For this review, take the finished solid that the model builds, in its own axes (mm). A direction names the side the tool comes from. Give positions to 0.01 mm unless a question says otherwise; leave off trailing zeros. Write each loop counter-clockwise with the first axis right and the second up, starting at its lowest first coordinate (ties: lowest second). Pieces come first, ordered by that corner, then holes.
1) We need section A-A on y = 1. Give the boundary of the cut face in (x, z), and give its area (3 significant figures).
2) Machinability: for faces 1 (the face through (125.556, -67, 2)), 2 (the face through (-121, 55.466, 2)), 3 (the face through (0, -40.914, 2)), 4 (the face through (121, -29.881, 2)), 5 (the face through (-41.016, 12, 2)), which of the approach directions +Z, -Z, +X, -X, +Y, -Y give a long, thin tool a straight path to every point of the face, cutting with its end or side? Answer none if there is none.
3) We need section B-B on x = 59. Give the boundary of the cut face in (y, z), and give its area (3 significant figures).
4) We need section D-D on x = -90. Give the boundary of the cut face in (y, z), and give its area (3 significant figures).
5) Wall thickness on line 1 along Y through (x, z) = (26.5, 0.55); line 2 along X through (y, z) = (39, 2.1); line 3 along Y through (x, z) = (-79.5, 2.9): over which ranges is each line inside the solid? List them lowest first.
6) We need section C-C on y = -59.5. Give the boundary of the cut face in (x, z), and give its area (3 significant figures).
7) Draft analysis for pull direction X (two halves, no side actions). For faces 6 (the face through (-115.712, 13, 2)), 7 (the face through (96.437, -75.828, 2.465)), 8 (the face through (41.016, 12, 2)), 9 (the face through (-98, -102.438, 2)), state which applies: pulls with the +X half, pulls with the -X half, needs draft (parallel to the pull), parting line crosses it, or undercut.
8) For P1, Ø1.5, axis at y = 8, z = 3, coming from the +X side, flat-tipped, find the tip position at first contact; note if it passes through.
from build123d import *

# Parameters (mm, degrees)
SKETCH1_R           = 2.153330351
SKETCH1_R_2         = 12.817442563
SKETCH1_W           = 33.838048367
SKETCH1_H           = 82.031632405
BOSS_EXTRUDE1_DEPTH = 5
SKETCH5_R           = 62
CUT_EXTRUDE3_DEPTH  = 5
SKETCH6_R           = 1.6
SKETCH6_R_2         = 2
CUT_EXTRUDE4_DEPTH  = 10
BOSS_EXTRUDE2_DEPTH = 5
CUT_EXTRUDE5_DEPTH  = 30


with BuildPart() as part:
    # Sketch1 → Boss-Extrude1 (new body)
    with BuildSketch(Plane.XY):
        with BuildLine():
            Line((125.53231807, 103.262634184), (91.381905468, 103.262634184))
            Line((91.381905468, 103.262634184), (77.913526918, 103.262634184))
            Line((77.913526918, 103.262634184), (36.253297751, 103.262634184))
            ThreePointArc((36.253297751, 103.262634184), (0, 93.454499378), (-36.253297751, 103.262634184))
            Line((-36.253297751, 103.262634184), (-77.913526918, 103.262634184))
            Line((-77.913526918, 103.262634184), (-91.381905468, 103.262634184))
            Line((-91.381905468, 103.262634184), (-125.53231807, 103.262634184))
            Line((-125.53231807, 103.262634184), (-125.54905558, 83.520799446))
            Line((-125.54905558, 83.520799446), (-125.554160174, 70.087177042))
            Line((-125.554160174, 70.087177042), (-125.554470078, 55.465919402))
            Line((-125.554470078, 55.465919402), (-115.83891891, 55.465919402))
            Line((-115.83891891, 55.465919402), (-115.711941884, 55.465919402))
            Line((-115.711941884, 55.465919402), (-115.711941884, 55.338942376))
            Line((-115.711941884, 55.338942376), (-115.711941884, -29.754151955))
            Line((-115.711941884, -29.754151955), (-115.711941884, -29.88112898))
            Line((-115.711941884, -29.88112898), (-115.83891891, -29.88112898))
            Line((-115.83891891, -29.88112898), (-125.555737773, -29.88112898))
            Line((-125.555737773, -29.88112898), (-125.555737773, -59.42445768))
            Line((-125.555737773, -59.42445768), (-125.555737773, -72.892836229))
            Line((-125.555737773, -72.892836229), (-125.555737773, -102.437610833))
            Line((-125.555737773, -102.437610833), (-101.198740966, -102.437610833))
            Line((-101.198740966, -102.437610833), (-87.730362416, -102.437610833))
            Line((-87.730362416, -102.437610833), (-70.522775483, -102.437610833))
            Line((-70.522775483, -102.437610833), (-52.513332124, -71.244339919))
            Line((-52.513332124, -71.244339919), (-47.927289793, -63.301081597))
            Line((-47.927289793, -63.301081597), (-35.002036695, -40.91388653))
            Line((-35.002036695, -40.91388653), (-5.325262411, -40.91388653))
            Line((-5.325262411, -40.91388653), (5.324834587, -40.91388653))
            Line((5.324834587, -40.91388653), (35.002036695, -40.91388653))
            Line((35.002036695, -40.91388653), (47.927289793, -63.301081597))
            Line((47.927289793, -63.301081597), (52.513332124, -71.244339919))
            Line((52.513332124, -71.244339919), (70.522775483, -102.437610833))
            Line((70.522775483, -102.437610833), (87.730362416, -102.437610833))
            Line((87.730362416, -102.437610833), (101.198740966, -102.437610833))
            Line((101.198740966, -102.437610833), (125.555737773, -102.437610833))
            Line((125.555737773, -102.437610833), (125.555737773, -72.892113277))
            Line((125.555737773, -72.892113277), (125.555737773, -59.423734727))
            Line((125.555737773, -59.423734727), (125.555737773, -29.88112898))
            Line((125.555737773, -29.88112898), (115.83891891, -29.88112898))
            ThreePointArc((115.83891891, -29.88112898), (115.749132594, -29.843938271), (115.711941884, -29.754151955))
            Line((115.711941884, -29.754151955), (115.711941884, 55.338942376))
            ThreePointArc((115.711941884, 55.338942376), (115.749132594, 55.428728692), (115.83891891, 55.465919402))
            Line((115.83891891, 55.465919402), (125.554470078, 55.465919402))
            Line((125.554470078, 55.465919402), (125.554160387, 70.077114789))
            Line((125.554160387, 70.077114789), (125.549047054, 83.530856147))
            Line((125.549047054, 83.530856147), (125.53231807, 103.262634184))
        make_face()
        with Locations((-101.032414216, -82.661089892)):
            Circle(SKETCH1_R, mode=Mode.SUBTRACT)
        with Locations((-90.522111314, -64.456711263)):
            Circle(SKETCH1_R_2, mode=Mode.SUBTRACT)
        with Locations((-80.011808412, -46.252332635)):
            Circle(SKETCH1_R, mode=Mode.SUBTRACT)
        with Locations((80.011808412, -46.252332635)):
            Circle(SKETCH1_R, mode=Mode.SUBTRACT)
        with Locations((90.522111314, -64.456711263)):
            Circle(SKETCH1_R_2, mode=Mode.SUBTRACT)
        with Locations((101.032414216, -82.661089892)):
            Circle(SKETCH1_R, mode=Mode.SUBTRACT)
        with Locations((57.934840386, 12.792395211)):
            Rectangle(SKETCH1_W, SKETCH1_H, mode=Mode.SUBTRACT)
        with Locations((-57.934840386, 12.792395211)):
            Rectangle(SKETCH1_W, SKETCH1_H, mode=Mode.SUBTRACT)
    extrude(amount=BOSS_EXTRUDE1_DEPTH)

    # Sketch5 → Cut-Extrude3 (cut)
    with BuildSketch(Plane.XY.offset(5)):
        with Locations((0, 135.292395211)):
            Circle(SKETCH5_R)
    extrude(amount=-CUT_EXTRUDE3_DEPTH, mode=Mode.SUBTRACT)

    # Sketch6 → Cut-Extrude4 (cut)
    with BuildSketch(Plane.XY.offset(5)):
        with Locations((26.464466094, 69.756861305)):
            Circle(SKETCH6_R)
        with Locations((26.464466094, 48.827929116)):
            Circle(SKETCH6_R)
        with Locations((-26.464466094, 69.756861305)):
            Circle(SKETCH6_R)
        with Locations((-26.464466094, 48.827929116)):
            Circle(SKETCH6_R)
        with Locations((-37.015816202, 30.292395211)):
            Circle(SKETCH6_R_2)
        with Locations((-37.015816202, -4.707604789)):
            Circle(SKETCH6_R_2)
        with Locations((-6.015816202, -4.707604789)):
            Circle(SKETCH6_R_2)
        with Locations((-6.015816202, 30.292395211)):
            Circle(SKETCH6_R_2)
        with Locations((6.015816202, 30.292395211)):
            Circle(SKETCH6_R_2)
        with Locations((6.015816202, -4.707604789)):
            Circle(SKETCH6_R_2)
        with Locations((37.015816202, 30.292395211)):
            Circle(SKETCH6_R_2)
        with Locations((37.015816202, -4.707604789)):
            Circle(SKETCH6_R_2)
    extrude(amount=-CUT_EXTRUDE4_DEPTH, mode=Mode.SUBTRACT)

    # Sketch8 → Boss-Extrude2 (add)
    with BuildSketch(Plane(origin=(0, 0, 0), x_dir=(-1, 0, 0), z_dir=(0, 0, -1))):
        with BuildLine():
            Line((-125.53231807, 103.262634184), (-125.53231807, 111.292395211))
            Line((-125.53231807, 111.292395211), (125.53231807, 111.292395211))
            Line((125.53231807, 111.292395211), (125.53231807, 103.262634184))
            Line((125.53231807, 103.262634184), (53.085726976, 103.262634184))
            ThreePointArc((53.085726976, 103.262634184), (0, 73.292395211), (-53.085726976, 103.262634184))
            Line((-53.085726976, 103.262634184), (-125.53231807, 103.262634184))
        make_face()
    extrude(amount=-BOSS_EXTRUDE2_DEPTH)

    # Sketch10 → Cut-Extrude5 (cut)
    with BuildSketch(Plane.XY.offset(5)):
        with BuildLine():
            Line((-30.5, 111.292395211), (-65.587998232, 111.292395211))
            ThreePointArc((-65.587998232, 111.292395211), (-51.367987693, 97.636707664), (-34.384510932, 87.624314384))
            ThreePointArc((-34.384510932, 87.624314384), (-32.452174676, 86.797991587), (-30.5, 86.01969421))
            Line((-30.5, 86.01969421), (-30.5, 111.292395211))
        make_face()
        with BuildLine():
            Line((65.587998232, 111.292395211), (30.5, 111.292395211))
            Line((30.5, 111.292395211), (30.5, 86.01969421))
            ThreePointArc((30.5, 86.01969421), (33.278602522, 87.144484688), (36.015816202, 88.366551325))
            ThreePointArc((36.015816202, 88.366551325), (52.079097115, 98.182018442), (65.587998232, 111.292395211))
        make_face()
    extrude(amount=-CUT_EXTRUDE5_DEPTH, mode=Mode.SUBTRACT)


solid = part.part
Results list:
1. outline: (-115.71, 0) - (-74.85, 0) - (-74.85, 5) - (-115.71, 5) - close; (-41.02, 0) - (41.02, 0) - (41.02, 5) - (-41.02, 5) - close; (74.85, 0) - (115.71, 0) - (115.71, 5) - (74.85, 5) - close
1. area: 819 mm2
2. face 1: +Z, -Z, +X, +Y, -Y
2. face 2: +Z, -Z, -X
2. face 3: +Z, -Z, -Y
2. face 4: +Z, -Z, +X
2. face 5: +Z, -Z
3. outline: (-82.48, 0) - (-28.22, 0) - (-28.22, 5) - (-82.48, 5) - close; (53.81, 0) - (104.17, 0) - (104.17, 5) - (53.81, 5) - close
3. area: 523 mm2
4. outline: (-102.44, 0) - (-77.26, 0) - (-77.26, 5) - (-102.44, 5) - close; (-51.65, 0) - (111.29, 0) - (111.29, 5) - (-51.65, 5) - close
4. area: 941 mm2
5. line 1: y = -40.91 to 47.23, 50.43 to 68.16, 71.36 to 111.29
5. line 2: x = -115.71 to -74.85, -41.02 to 41.02, 74.85 to 115.71
5. line 3: y = -102.44 to -71, -57.91 to -48.34, -44.16 to 111.29
6. outline: (-125.56, 0) - (-102.34, 0) - (-102.34, 5) - (-125.56, 5) - close; (-78.7, 0) - (-45.73, 0) - (-45.73, 5) - (-78.7, 5) - close; (45.73, 0) - (78.7, 0) - (78.7, 5) - (45.73, 5) - close; (102.34, 0) - (125.56, 0) - (125.56, 5) - (102.34, 5) - close
6. area: 562 mm2
7. face 6: pulls with the -X half
7. face 7: undercut
7. face 8: undercut
7. face 9: needs draft
8. P1: stops at x = 115.71
